Verification items for the finished model (mm, model axes). A direction names the side the tool comes from. Round coordinates to 2 decimals unless told otherwise and drop trailing zeros. Write each loop counter-clockwise with the first axis right and the second up, starting at its lowest first coordinate (ties: lowest second). Pieces come first, ordered by that corner, then holes. Notation, with made-up numbers: (23, -17) - (35, -17) arc R17 ccw to (35, 1) - close; hole circle Ø3 at (34, -36). An arc over 180 degrees is marked (long way). Write each question's results on one line, items separated by ' | '.
```python
from build123d import *

# Parameters (mm, degrees)
ESQUISSE1_W             = 112
ESQUISSE1_H             = 8
BOSS_EXTRU_1_DEPTH      = 450.3
ENL_V_MAT_EXTRU_1_DEPTH = 10
ESQUISSE3_W             = 40
ESQUISSE3_H             = 8
BOSS_EXTRU_2_DEPTH      = 8
ESQUISSE4_R             = 35
ENL_V_MAT_EXTRU_2_DEPTH = 10
ESQUISSE5_W             = 8
ESQUISSE5_H             = 60
BOSS_EXTRU_3_DEPTH      = 8
BOSS_EXTRU_5_DEPTH      = 8
CONG_1_R                = 10
ESQUISSE8_R             = 2.6
ENL_V_MAT_EXTRU_3_DEPTH = 8
ESQUISSE9_R             = 10
ENL_V_MAT_EXTRU_4_DEPTH = 10


with BuildPart() as part:
    # Esquisse1 → Boss.-Extru.1 (new body)
    with BuildSketch(Plane.XY):
        with Locations((-92, -52)):
            Rectangle(ESQUISSE1_W, ESQUISSE1_H)
    extrude(amount=BOSS_EXTRU_1_DEPTH)

    # Esquisse2 → Enlèv. mat.-Extru.1 (cut)
    with BuildSketch(Plane.XZ.offset(56)):
        Polygon((-148, 360.15), (-138, 350.15), (-138, 100.15), (-148, 90.15), align=None)
    extrude(amount=-ENL_V_MAT_EXTRU_1_DEPTH, mode=Mode.SUBTRACT)

    # Esquisse3 → Boss.-Extru.2 (add)
    with BuildSketch(Plane.XZ.offset(56)):
        with Locations((-92, 454.3)):
            Rectangle(ESQUISSE3_W, ESQUISSE3_H)
        with Locations((-92, -4)):
            Rectangle(ESQUISSE3_W, ESQUISSE3_H)
    extrude(amount=-BOSS_EXTRU_2_DEPTH)

    # Esquisse4 → Enlèv. mat.-Extru.2 (cut)
    with BuildSketch(Plane(origin=(0, -48, 0), x_dir=(1, 0, 0), z_dir=(0, 1, 0))):
        with Locations(Location((-108, -50, 0), (0, 0, 180))):
            Circle(ESQUISSE4_R)
        with Locations(Location((-108, -400.3, 0), (0, 0, 180))):
            Circle(ESQUISSE4_R)
    extrude(amount=-ENL_V_MAT_EXTRU_2_DEPTH, mode=Mode.SUBTRACT)

    # Esquisse5 → Boss.-Extru.3 (add)
    with BuildSketch(Plane.XZ.offset(56)):
        with Locations((-32, 225.3)):
            Rectangle(ESQUISSE5_W, ESQUISSE5_H)
        with Locations((-32, 375.3)):
            Rectangle(ESQUISSE5_W, ESQUISSE5_H)
        with Locations((-32, 75.3)):
            Rectangle(ESQUISSE5_W, ESQUISSE5_H)
    extrude(amount=-BOSS_EXTRU_3_DEPTH)

    # Esquisse7 → Boss.-Extru.5 (add)
    with BuildSketch(Plane.XZ.offset(56)):
        with BuildLine():
            Line((-148, 438.049172176), (-148, 362.550827824))
            ThreePointArc((-148, 362.550827824), (-163, 400.3), (-148, 438.049172176))
        make_face()
        with BuildLine():
            Line((-148, 12.250827824), (-148, 87.749172176))
            ThreePointArc((-148, 87.749172176), (-163, 50), (-148, 12.250827824))
        make_face()
    extrude(amount=-BOSS_EXTRU_5_DEPTH)

    # Congé1
    cong_1_edges = [part.edges().sort_by_distance(p)[0] for p in [
        (-148, -52, 0),
        (-148, -52, 450.3),
    ]]
    fillet(cong_1_edges, radius=CONG_1_R)

    # Esquisse8 → Enlèv. mat.-Extru.3 (cut)
    with BuildSketch(Plane(origin=(0, -48, 0), x_dir=(1, 0, 0), z_dir=(0, 1, 0))):
        with Locations(Location((-51, -142.3, 0), (0, 0, 270))):
            Circle(ESQUISSE8_R)
        with Locations(Location((-51, -164.3, 0), (0, 0, 270))):
            Circle(ESQUISSE8_R)
        with Locations(Location((-51, -312.3, 0), (0, 0, 270))):
            Circle(ESQUISSE8_R)
        with Locations(Location((-51, -290.3, 0), (0, 0, 270))):
            Circle(ESQUISSE8_R)
    extrude(amount=-ENL_V_MAT_EXTRU_3_DEPTH, mode=Mode.SUBTRACT)

    # Esquisse9 → Enlèv. mat.-Extru.4 (cut)
    with BuildSketch(Plane.XZ.offset(56)):
        with Locations((-71, 305.15)):
            Circle(ESQUISSE9_R)
        with Locations((-71, 275.15)):
            Circle(ESQUISSE9_R)
        with Locations((-71, 245.15)):
            Circle(ESQUISSE9_R)
    extrude(amount=-ENL_V_MAT_EXTRU_4_DEPTH, mode=Mode.SUBTRACT)


solid = part.part
```
(1) Section check B-B (x = -108). Record the cut outline in (y, z), plus the area to 3 significant figures.
Answer:
outline: (-56, -8) - (-48, -8) - (-48, 15) - (-56, 15) - close; (-56, 85) - (-48, 85) - (-48, 365.3) - (-56, 365.3) - close; (-56, 435.3) - (-48, 435.3) - (-48, 458.3) - (-56, 458.3) - close | area: 2,610 mm2
(2) Section check D-D (y = -54). State how many separate pieces and enclosed holes the cut face has, plus the area to 3 significant figures.
Answer:
separate pieces: 1 | enclosed holes: 9 | area: 42,700 mm2
(3) Mould release check, pull along Z, two halves, no side actions. Record for faces 1 (the flat face through (-54, -52, 450.3)), 2 (the flat face through (-72, -52, 454)), 3 (the flat face through (-143.07, -52.06, 355.22)): released by +Z, released by -Z, zero draft, split by the parting line, or undercut.
Answer:
face 1: released by +Z | face 2: zero draft | face 3: undercut
(4) Set-up check for faces 4 (the flat face through (-112, -52, 454)), 5 (the flat face through (-36, -52, 22)), 6 (the flat face through (-32, -52, 195.3)): record each of +Z, -Z, +X, -X, +Y, -Y from which the full face is reachable in a straight line by a thin tool's end or side.
Answer:
face 4: +Z, -X, +Y, -Y | face 5: -Z, +X, +Y, -Y | face 6: +X, +Y, -Y
(5) Go/stop test with flat-tipped pins: pin 1 Ø2.5 at (x, y) = (-33, -50.5) entering from +Z; pin 2 Ø1.8 at (y, z) = (-54, 11) entering from -X; pin 3 Ø4 at (y, z) = (-51.5, -5.5) entering from -X. Record where each tip stops, or that it passes through.
Answer:
pin 1: z = 405.3 | pin 2: x = -148 | pin 3: x = -112
(6) Section check C-C (z = 72.5). Record the cut outline in (x, y).
Answer:
outline: (-158.19, -56) - (-134.81, -56) - (-134.81, -48) - (-158.19, -48) - close; (-81.19, -56) - (-28, -56) - (-28, -48) - (-81.19, -48) - close
(7) Section check A-A (z = 400.3). Record the cut outline in (x, y), plus the area to 3 significant figures.
Answer:
outline: (-163, -56) - (-143, -56) - (-143, -48) - (-163, -48) - close; (-73, -56) - (-28, -56) - (-28, -48) - (-73, -48) - close | area: 520 mm2
(8) Thickness scan on L1, parallel to Z at x = -108, y = -52; L2, parallel to Z at x = -71, y = -53; L3, parallel to X at y = -51.75, z = 164.3. Record the ranges inside material, lowest first.
Answer:
L1: -8 to 15, 85 to 365.3, 435.3 to 458.3 | L2: 0 to 235.15, 255.15 to 265.15, 285.15 to 295.15, 315.15 to 450.3 | L3: -138 to -53.6, -48.4 to -36
